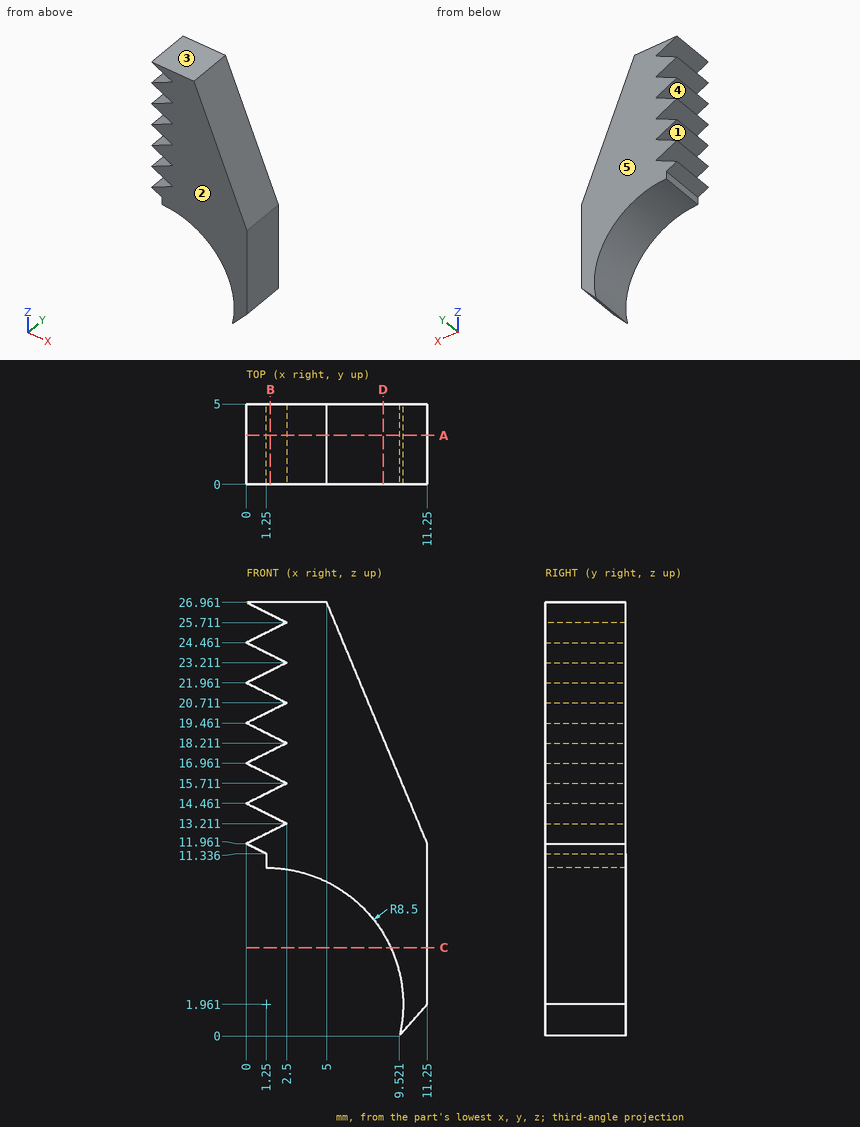
The drawing under review shows one solid part. Ordinate dimensions are in mm from its lowest x, y, z. A direction names the side the tool comes from. Coordinates: 2 decimals unless noted, no trailing zeros. Write each loop counter-clockwise with the first axis right and the second up, starting at its lowest first coordinate (ties: lowest second). Pieces come first, ordered by that corner, then holes. Notation, with made-up numbers: (60.25, 73.25) - (94.25, 73.25) arc R13 ccw to (94.25, 79.25) - close; hole circle Ø10 at (64, -34). An arc over 180 degrees is marked (long way). Answer in a Markdown table with one row per item. Add a question column.
Q1. For probe 1 along X at (y, z) = (4.1, 10.75); probe 2 along Z at (x, y) = (6.75, 3.3); probe 3 along Z at (x, y) = (3.5, 0.8), list the stretches that pass through material, from the lowest coordinate up.
Q2. For P1, Ø1.5, axis at x = 5, z = 24, coming from the -Y side; P2, Ø1.5, axis at x = 6.5, y = 3, coming from the -Z side; P3, Ø1, axis at y = 1, z = 20.5, coming from the +X side, all flat-tipped, find the tip position at first contact; note any pin that passes through.
Q3. We need section B-B, the plane x = 1.5. State the section outline as (y, z) points.
Q4. Tool access review of the marked faces 4 and 5: name each direction out of +Z, -Z, +X, -X, +Y, -Y from which nothing blocks a thin tool from reaching the whole face with its end or side.
Q5. We need section C-C, the plane z = 5.5. State the section outline as (x, y) points.
Q6. We need section D-D, the plane x = 8.5. State the section outline as (y, z) points, and give its area (3 significant figures).
Q7. Draft analysis for pull direction Z (two halves, no side actions). For the marked faces 1, 2 and 3, state which applies: +Z half, -Z half, draft (parallel to the pull), parting line (faces both ways), or undercut.
Q8. We need section A-A, the plane y = 3.05. State the section outline as (x, z) points.
Answer list:
| question | item | result |
|---|---|---|
| 1 | probe 1 | x = 1.25 to 11.25 |
| 1 | probe 2 | z = 8.44 to 22.76 |
| 1 | probe 3 | z = 10.16 to 26.96 |
| 2 | P1 | stops at y = 0 |
| 2 | P2 | stops at z = 7.98 |
| 2 | P3 | stops at x = 7.9 |
| 3 | outline | (0, 10.46) - (5, 10.46) - (5, 12.71) - (0, 12.71) - close; (0, 13.71) - (5, 13.71) - (5, 15.21) - (0, 15.21) - close; (0, 16.21) - (5, 16.21) - (5, 17.71) - (0, 17.71) - close; (0, 18.71) - (5, 18.71) - (5, 20.21) - (0, 20.21) - close; (0, 21.21) - (5, 21.21) - (5, 22.71) - (0, 22.71) - close; (0, 23.71) - (5, 23.71) - (5, 25.21) - (0, 25.21) - close; (0, 26.21) - (5, 26.21) - (5, 26.96) - (0, 26.96) - close |
| 4 | face 4 | -X, +Y, -Y |
| 4 | face 5 | +Z, -Z, +X, -X, +Y |
| 5 | outline | (8.98, 0) - (11.25, 0) - (11.25, 5) - (8.98, 5) - close |
| 6 | outline | (0, 6.4) - (5, 6.4) - (5, 18.56) - (0, 18.56) - close |
| 6 | area | 60.8 mm2 |
| 7 | face 1 | undercut |
| 7 | face 2 | draft |
| 7 | face 3 | +Z half |
| 8 | outline | (0, 11.96) - (1.25, 11.34) - (1.25, 10.46) arc R8.5 cw to (9.52, 0) - (11.25, 1.96) - (11.25, 11.96) - (5, 26.96) - (0, 26.96) - (2.5, 25.71) - (0, 24.46) - (2.5, 23.21) - (0, 21.96) - (2.5, 20.71) - (0, 19.46) - (2.5, 18.21) - (0, 16.96) - (2.5, 15.71) - (0, 14.46) - (2.5, 13.21) - close |
